from build123d import *

# Parameters (mm, degrees)
EXTRUDE_419_DEPTH   = 20
SKETCH1_R           = 25
BOSS_EXTRUDE1_DEPTH = 30
SKETCH2_R           = 20
CUT_EXTRUDE1_DEPTH  = 119.427186528


with BuildPart() as part:
    # Эскиз1 → Extrude 419 (new body)
    with BuildSketch(Plane(origin=(0, 0, 0), x_dir=(-1, 0, 0), z_dir=(0, -1, 0))):
        with BuildLine():
            Line((-78.917505692, 23.388614652), (-17.835027079, 46.710938859))
            ThreePointArc((-17.835027079, 46.710938859), (-0.148812417, 49.999778548), (17.556665634, 46.816273793))
            Line((17.556665634, 46.816273793), (78.776887546, 23.857954408))
            ThreePointArc((78.776887546, 23.857954408), (94.998038561, 0.610466623), (79.076996078, -22.84357002))
            Line((79.076996078, -22.84357002), (18.156882698, -46.586775062))
            ThreePointArc((18.156882698, -46.586775062), (0.148812417, -49.999778548), (-17.879254632, -46.694028031))
            Line((-17.879254632, -46.694028031), (-78.939619469, -23.313868793))
            ThreePointArc((-78.939619469, -23.313868793), (-94.99998935, 0.044982802), (-78.917505692, 23.388614652))
        make_face()
    extrude(amount=EXTRUDE_419_DEPTH)

    # Sketch1 → Boss-Extrude1 (add)
    with BuildSketch(Plane.XZ.offset(20)):
        with Locations(Location((0, 0, 0), (0, 0, 270))):
            Circle(SKETCH1_R)
    extrude(amount=BOSS_EXTRUDE1_DEPTH)

    # Sketch2 → Cut-Extrude1 (cut, through all)
    with BuildSketch(Plane.XZ.offset(50)):
        with Locations(Location((0, 0, 0), (0, 0, 270))):
            Circle(SKETCH2_R)
    extrude(amount=-CUT_EXTRUDE1_DEPTH, mode=Mode.SUBTRACT)


solid = part.part
Could you check a few things on this model? Use its own coordinates, in mm. A direction names the side the tool comes from. Coordinates: 2 decimals unless noted, no trailing zeros. Order: outer loops, then holes, each group sorted by start corner. A loop starts at its lowest first (then second) coordinate and runs counter-clockwise, first axis right, second up. Notation, with made-up numbers: (0, 48) - (55, 48) arc R31 cw to (55, 77) - close; hole circle Ø3 at (83.5, -13). An arc over 180 degrees is marked (long way). Answer in a Markdown table with one row per item. Add a question column.
(1) If we section it at A-A, the plane x = 0: Please give me the cut outline in (y, z), then the cut area to 3 significant figures.
(2) If we mould it in two halves opening along Z, with no side actions, what happens to faces 1 (the face through (-94.99, -9.86, -1.03)), 2 (the face through (-19.524, -25.35, 4.336)), 3 (the face through (0, -10, -50))? For each: released by +Z, released by -Z, zero draft, split by the parting line, or undercut.
(3) If we section it at C-C, the plane z = -5: Please give me the cut outline in (x, y).
(4) I need wall thicknesses on L1, parallel to X at y = -12, z = 0; L2, parallel to X at y = -38, z = 0; L3, parallel to Y at x = -2.5, z = -36. Which ranges of each line are inside material? Lowest first, please.
(5) If we section it at D-D, the plane z = 29.5: Please give me the cut outline in (x, y).
(6) If we section it at B-B, the plane y = -13: Please give me the cut outline in (x, z), then the cut area to 3 significant figures.
(7) Will these pins go through, and if not, where does the flat tip stop? pin 1 (6 mm diameter, centred on y = -30, z = 5.5, fed in from +X); pin 2 (8 mm diameter, centred on y = -35.5, z = 20, fed in from -X); pin 3 (8 mm diameter, centred on y = -45, z = 3.5, fed in from -X).
(8) On a 3-axis mill with a long thin cutter (end or side, diameter ignored), from which of +Z, -Z, +X, -X, +Y, -Y can I reach the whole of each face in a straight line? I mean faces 4 (the face through (7.509, -34.79, -23.846)), 5 (the face through (95, -10, 0)). Say none if no direction works.
Results are:
| question | item | result |
|---|---|---|
| 1 | outline | (-50, -25) - (-20, -25) - (-20, -50) - (0, -50) - (0, -20) - (-50, -20) - close; (-50, 20) - (0, 20) - (0, 50) - (-20, 50) - (-20, 25) - (-50, 25) - close |
| 1 | area | 1,500 mm2 |
| 2 | face 1 | split by the parting line |
| 2 | face 2 | undercut |
| 2 | face 3 | released by -Z |
| 3 | outline | (-94.58, -20) - (-24.49, -20) - (-24.49, -50) - (-19.36, -50) - (-19.36, 0) - (-94.58, 0) - close; (19.36, -50) - (24.49, -50) - (24.49, -20) - (94.5, -20) - (94.5, 0) - (19.36, 0) - close |
| 4 | L1 | x = -94.99 to -20, 20 to 95 |
| 4 | L2 | x = -25 to -20, 20 to 25 |
| 4 | L3 | y = -20 to 0 |
| 5 | outline | (-62, -20) - (62.78, -20) - (62.78, 0) - (-62, 0) - close |
| 6 | outline | (-79.08, 22.84) arc R25 ccw to (-78.78, -23.86) - (-17.56, -46.82) arc R50 ccw to (17.84, -46.71) - (78.92, -23.39) arc R25 ccw to (78.94, 23.31) - (17.88, 46.69) arc R50 ccw to (-18.16, 46.59) - close; hole circle Ø40 at (0, 0) |
| 6 | area | 11,900 mm2 |
| 7 | pin 1 | stops at x = 24.87 |
| 7 | pin 2 | stops at x = -19.21 |
| 7 | pin 3 | stops at x = -25 |
| 8 | face 4 | -Y |
| 8 | face 5 | +X, +Y, -Y |
